The listing builds one solid part. Answer for the finished solid, in the listing's coordinates (mm). Coordinates: 2 decimals unless noted, no trailing zeros. Write each loop counter-clockwise with the first axis right and the second up, starting at its lowest first coordinate (ties: lowest second). Pieces come first, ordered by that corner, then holes. Notation, with made-up numbers: M 1,-9 L 44,-9 A20 ccw 44,8 Z; hole C 7,46 d4. An arc over 180 degrees is marked long. Put each result on its own line as item: value. Start each with the question number.
Solid Edge part; units mm, degrees
sketch "Sketch1" plane through (0, 0, 0) normal (0, 0, 1) x (1, 0, 0)
  line L0 (0.2011, -9.998) -> (-9.3087, -3.6535)
  arc A0 (-9.3087, -3.6535) -> (0.2011, -9.998) centre (0, 0) cw
  line L1 (-1.4897, 3.2779) -> (3.5986, -0.1168)
  arc A1 (3.5986, -0.1168) -> (-1.4897, 3.2779) centre (0, 0) cw
extrude "Protrusion1" add sketch "Sketch1" along normal blind 12
sketch "Sketch2" plane through (-0.8973, 0, 0) normal (0, 0, -1) x (0, -1, 0)
  line L0 (9.998, -1.0984) -> (3.6535, 8.4114)
  line L1 (3.6535, 8.4114) -> (8.0376, 19.5818)
  line L2 (9.998, -1.0984) -> (21.9956, -1.3398)
  arc A0 (8.0376, 19.5818) -> (21.9956, -1.3398) centre (0, -0.8973) ccw
  arc A1 (0.1168, -4.4959) -> (-3.2779, 0.5923) centre (0, -0.8973) ccw
  line L3 (-3.2779, 0.5923) -> (0.1168, -4.4959)
extrude "ExtrudedProtrusion_2" add sketch "Sketch2" along normal blind 1.5
sketch "Sketch3" plane through (0, 0.0022, -1.5) normal (0, 0, -1) x (0.0201117, -0.9997977, 0)
  arc A0 (8.4391, -5.3682) -> (10.0022, 0) centre (0.0022, 0) ccw
  line L0 (10.0022, 0) -> (3.4677, 9.3804)
  arc A1 (3.4677, 9.3804) -> (-0.8212, 9.9661) centre (0.0022, 0) ccw
  line L1 (-0.8212, 9.9661) -> (-1.8094, 21.9253)
  arc A2 (-1.8094, 21.9253) -> (19.3291, -10.5105) centre (0.0022, 0) cw
  line L2 (8.4391, -5.3682) -> (19.3291, -10.5105)
extrude "ExtrudedCutout_1" cut sketch "Sketch3" against normal blind 22.4982
1) A cutting plane is placed at C-C on y = -5.5. Write down the section's boundary in (x, z).
2) A cutting plane is placed at B-B on y = -1. Write down the section's boundary in (x, z).
3) A cutting plane is placed at D-D on x = -17. Write down the section's boundary in (y, z).
4) A cutting plane is placed at A-A on z = 9.25. Write down the section's boundary in (x, y), then the cut area to 3 significant figures.
5) Determine the mould class of faces 1 (the face through (-1.91, -3.05, 5.92)), 2 (the face through (12.174, 18.325, -0.74)), 3 (the face through (-16, 1, -1)), 4 (the face through (5, 11, 0)) for opening direction X: +X half, -X half, draft (parallel to the pull), parting line (faces both ways), or undercut.
6) Straight lines are drawn through the part: probe 1 along Y at (x, z) = (0, 4.5); probe 2 along X at (y, z) = (0, -0.95); probe 3 along Y at (x, z) = (0, -0.5). For each, find the intervals that lie inside material, in ascending order.
7) Given pin 1 Ø5 at (x, z) = (-8.5, 10) entering from +Y; pin 2 Ø1.5 at (y, z) = (8.5, 5.5) entering from -X; pin 3 Ø1.5 at (x, z) = (-4, 9.5) entering from +Y, each flat-ended and moving along its own axis, determine where each tip first touches the part or whether it passes through.
Answers follow:
1. outline: M -6.54,-1.5 L 21.3,-1.5 L 21.3,0 L 8.35,0 L 8.35,12 L -6.54,12 Z
2. outline: M -9.95,-1.5 L -3.46,-1.5 L -3.46,12 L -9.95,12 Z; M 3.46,-1.5 L 21.98,-1.5 L 21.98,0 L 9.95,0 L 9.95,12 L 3.46,12 Z
3. outline: M 1.06,-1.5 L 13.96,-1.5 L 13.96,0 L 1.06,0 Z
4. outline: M -9.31,-3.65 L 0.2,-10 A10 ccw long Z; hole M -1.49,3.28 A3.6 ccw long 3.6,-0.12 Z
4. area: 267 mm²
5. face 1: undercut
5. face 2: parting line
5. face 3: -X half
5. face 4: draft
6. probe 1: y = -9.86 to -3.6, 2.28 to 10
6. probe 2: x = -10 to -3.6, 3.42 to 22
6. probe 3: y = -9.86 to -3.6, 2.28 to 22
7. pin 1: stops at y = 8
7. pin 2: stops at x = -6.32
7. pin 3: stops at y = 9.46
